Here's the drawing with two shaded views (mm, measured from the low corner). I have some questions. Coordinates: 2 decimals unless noted, no trailing zeros. Loops run counter-clockwise (first coordinate to the right, second up) from the corner with the lowest first, then second, coordinate; pieces in that order, holes last. Notation, with made-up numbers: M 3.25,51 L 22.25,51 A25 ccw 22.25,79 Z; hole C -30,-27.5 d4. An arc over 180 degrees is marked long. Use one line per item in the form item = value. Start each with the question number.
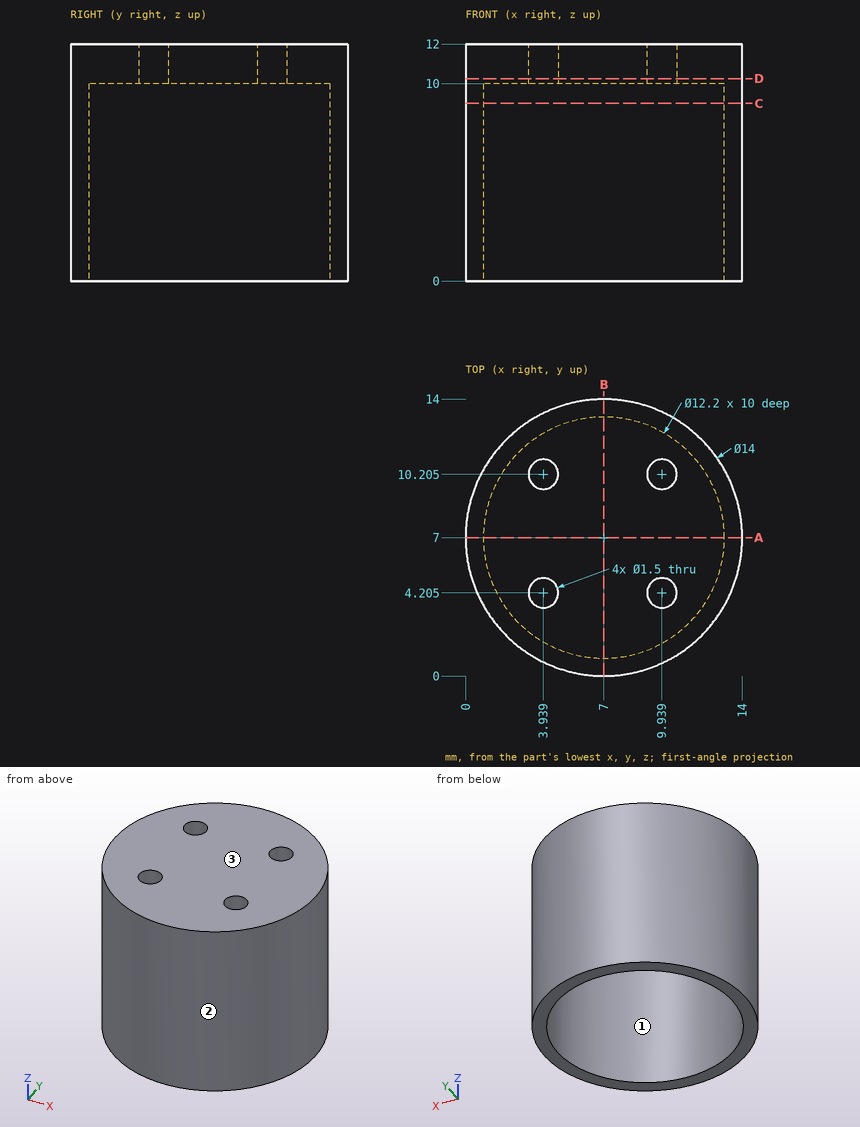
Item 1: I want a section at D-D (z = 10.25). Count the separate pieces of the cut face and the enclosed holes in it, plus the area to 3 significant figures.
Item 2: I'm going to push flat-ended pins straight in: P1, Ø6, axis at x = 9.5, y = 8.5, coming from the -Z side; P2, Ø1.2, axis at x = 9.94, y = 4.2, coming from the -Z side; P3, Ø4, axis at y = 11.5, z = 6.5, coming from the -X side. Where does each tip first touch, or does it pass through?
Item 3: I want a section at C-C (z = 9). Write out the boundary of the cut face in (x, y).
Item 4: Please list where these lines run through material, in increasing order: line 1 along Y through (x, z) = (6.75, 8.5) (1 decimal); line 2 along X through (y, z) = (10.75, 11.25) (1 decimal); line 3 along Z through (x, y) = (7, 12.5).
Item 5: I want a section at A-A (y = 7). Write out the boundary of the cut face in (x, z).
Item 6: Thinking about a two-plate mould opening in Y: for the marked faces 1, 2 and 3, which applies, pulls with the +Y half, pulls with the -Y half, needs draft (parallel to the pull), parting line crosses it, or undercut?
Worked answers:
q1.separate_pieces = 1
q1.enclosed_holes = 4
q1.area = 147 mm²
q2.P1 = 10
q2.P2 = through
q2.P3 = 0.46
q3.outline = C 7,7 d14; hole C 7,7 d12.2
q4.line_1 = 0 to 0.9, 13.1 to 14
q4.line_2 = 1.1 to 3.4, 4.5 to 9.4, 10.5 to 12.9
q4.line_3 = 10 to 12
q5.outline = M 0,0 L 0.9,0 L 0.9,10 L 13.1,10 L 13.1,0 L 14,0 L 14,12 L 0,12 Z
q6.face_1 = undercut
q6.face_2 = parting line crosses it
q6.face_3 = needs draft
